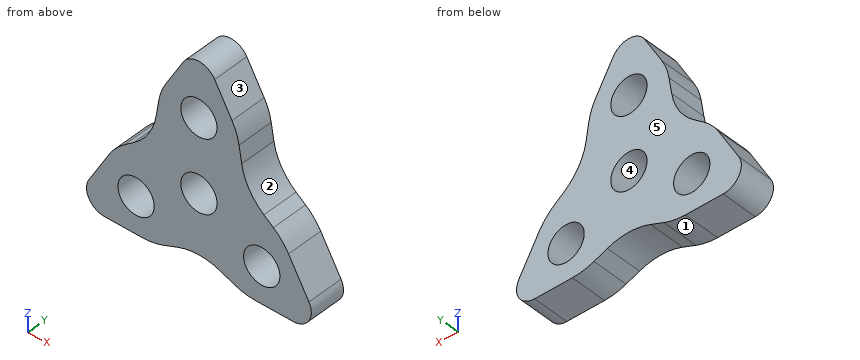
from build123d import *

# Parameters (mm, degrees)
F0_R     = 12.7
F1_DEPTH = 25.4
F3_DEPTH = 25.4
F4_R     = 12.7
F5_R     = 40.64


with BuildPart() as f1:
    # F0 (on Front) → F1 (new body)
    with BuildSketch(Plane.XZ):
        Polygon((0, 101.6), (-87.9881810245, -50.8), (87.9881810245, -50.8), align=None)
        with Locations((-43.9940905122, -25.4)):
            Circle(F0_R, mode=Mode.SUBTRACT)
        Circle(F0_R, mode=Mode.SUBTRACT)
        with Locations((43.9940905122, -25.4)):
            Circle(F0_R, mode=Mode.SUBTRACT)
        with Locations((0, 50.8)):
            Circle(F0_R, mode=Mode.SUBTRACT)
    extrude(amount=F1_DEPTH)

    # F2 (on face) → F3 (cut)
    with BuildSketch(Plane.XZ.offset(25.4)):
        Polygon((-32.5348633552, 19.8479636515), (-26.9087873497, 54.9926131403), (-58.6587873497, 0), align=None)
        Polygon((58.6587873497, 0), (26.9087873497, 54.9926131403), (32.5348633552, 19.8479636515), align=None)
        Polygon((0, -38.1), (-31.75, -50.8), (31.75, -50.8), align=None)
    extrude(amount=-F3_DEPTH, mode=Mode.SUBTRACT)

    # F4
    f4_edges = [f1.edges().sort_by_distance(p)[0] for p in [
        (0, -12.7, 101.6),
        (-87.988181, -12.7, -50.8),
        (87.988181, -12.7, -50.8),
    ]]
    fillet(f4_edges, radius=F4_R)

    # F5
    f5_edges = [f1.edges().sort_by_distance(p)[0] for p in [
        (-26.908787, -12.7, 54.992613),
        (-32.534863, -12.7, 19.847964),
        (-58.658787, -12.7, 0),
        (26.908787, -12.7, 54.992613),
        (32.534863, -12.7, 19.847964),
        (58.658787, -12.7, 0),
        (31.75, -12.7, -50.8),
        (0, -12.7, -38.1),
        (-31.75, -12.7, -50.8),
    ]]
    fillet(f5_edges, radius=F5_R)


solid = f1.part
Geometry check sheet. Reference: the model listing, model coordinates, mm. Face numbers are marked on the shaded views. A direction names the side the tool comes from. Round coordinates to 2 decimals unless told otherwise and drop trailing zeros. Order: outer loops, then holes, each group sorted by start corner. A loop starts at its lowest first (then second) coordinate and runs counter-clockwise, first axis right, second up. Notation, with made-up numbers: M 36.5,43 L 95.5,43 A34 ccw 95.5,80 Z; hole C -28.5,32.5 d1. An arc over 180 degrees is marked long. Answer in a Markdown table with one row per item. Add a question column.
Item 1: Sectioned sample at C-C, the plane y = -15.5. Enter the section's corners in (x, z).
Item 2: Sectioned sample at D-D, the plane x = -34. Enter the section's corners in (y, z), plus the area to 3 significant figures.
Item 3: Draft check along X on the marked faces 3, 4 and 5. Enter one of: released by +X, released by -X, zero draft, split by the parting line, or undercut.
Item 4: Depth check by flat-ended pin: pin 1 Ø1.5 at (x, y) = (3.5, -22.5) entering from -Z; pin 2 Ø6 at (x, y) = (-61, -12) entering from +Z; pin 3 Ø23 at (x, z) = (43.99, -25.4) entering from +Y; pin 4 Ø3 at (x, y) = (-53.5, -16.5) entering from +Z. Enter the tip coordinate at first touch or a pass-through.
Item 5: Sectioned sample at B-B, the plane z = 50.8. Enter the section's corners in (x, y), plus the area to 3 significant figures.
Item 6: Material ranges on L1, parallel to Z at x = -7.5, y = -9; L2, parallel to X at y = -7, z = -34; L3, parallel to Z at x = 6.5, y = -17, recorded low to high. Write a range as [from, to].
Item 7: Set-up check for the marked faces 1 and 2: record each of +Z, -Z, +X, -X, +Y, -Y from which the full face is reachable in a straight line by a thin tool's end or side.
Item 8: Sectioned sample at A-A, the plane x = 0. Enter the section's corners in (y, z).
Filled in:
| question | item | result |
|---|---|---|
| 1 | outline | M -76.99,-31.75 A12.7 ccw -65.99,-50.8 L -39.58,-50.8 A40.64 ccw -24.48,-47.89 L -15.09,-44.14 A40.64 cw 15.09,-44.14 L 24.48,-47.89 A40.64 ccw 39.58,-50.8 L 65.99,-50.8 A12.7 ccw 76.99,-31.75 L 62.75,-7.09 A40.64 ccw 52.14,4.95 L 45.5,9.99 A40.64 cw 29.96,35.93 L 28.09,47.59 A40.64 ccw 23.16,61.49 L 11,82.55 A12.7 ccw -11,82.55 L -23.16,61.49 A40.64 ccw -28.09,47.59 L -29.96,35.93 A40.64 cw -45.5,9.99 L -52.14,4.95 A40.64 ccw -62.75,-7.09 Z; hole C -43.99,-25.4 d25.4; hole C 0,0 d25.4; hole C 0,50.8 d25.4; hole C 43.99,-25.4 d25.4 |
| 2 | outline | M -25.4,-50.42 L 0,-50.42 L 0,-33.24 L -25.4,-33.24 Z; M -25.4,-17.56 L 0,-17.56 L 0,23.67 L -25.4,23.67 Z |
| 2 | area | 1,480 mm² |
| 3 | face 3 | released by +X |
| 3 | face 4 | undercut |
| 3 | face 5 | zero draft |
| 4 | pin 1 | stops at z = -41.45 |
| 4 | pin 2 | stops at z = -0.49 |
| 4 | pin 3 | passes through |
| 4 | pin 4 | stops at z = 5.06 |
| 5 | outline | M -27.45,-25.4 L -12.7,-25.4 L -12.7,0 L -27.45,0 Z; M 12.7,-25.4 L 27.45,-25.4 L 27.45,0 L 12.7,0 Z |
| 5 | area | 749 mm² |
| 6 | L1 | z = [-41.93, -10.25], [10.25, 40.55], [61.05, 86.45] |
| 6 | L2 | x = [-78.01, -53.34], [-34.65, 34.65], [53.34, 78.01] |
| 6 | L3 | z = [-41.75, -10.91], [10.91, 39.89], [61.71, 87.11] |
| 7 | face 1 | -Z, +Y, -Y |
| 7 | face 2 | +Z, +X, +Y, -Y |
| 8 | outline | M -25.4,-41.23 L 0,-41.23 L 0,-12.7 L -25.4,-12.7 Z; M -25.4,12.7 L 0,12.7 L 0,38.1 L -25.4,38.1 Z; M -25.4,63.5 L 0,63.5 L 0,88.9 L -25.4,88.9 Z |
